```python
from build123d import *

# Parameters (mm, degrees)
SKETCH_1_W          = 15
SKETCH_1_H          = 15
SKETCH_1_W_2        = 12
SKETCH_1_H_2        = 12
EXTRUDE_1_DEPTH     = 220
SKETCH_2_R          = 1.6
CUT_EXTRUDE_1_DEPTH = 221.638278637
SKETCH_3_R          = 1.6
CUT_EXTRUDE_2_DEPTH = 221.638278637


with BuildPart() as part:
    # ｽｹｯﾁ1 → ﾎﾞｽ - 押し出し1 (new body)
    with BuildSketch(Plane(origin=(0, 0, 0), x_dir=(0, 0, -1), z_dir=(1, 0, 0))):
        Rectangle(SKETCH_1_W, SKETCH_1_H)
        Rectangle(SKETCH_1_W_2, SKETCH_1_H_2, mode=Mode.SUBTRACT)
    extrude(amount=EXTRUDE_1_DEPTH)

    # ｽｹｯﾁ2 → ｶｯﾄ - 押し出し1 (cut, through all)
    with BuildSketch(Plane(origin=(0, 7.5, 0), x_dir=(1, 0, 0), z_dir=(0, 1, 0))):
        with Locations(Location((66.961524227, 0, 0), (0, 0, 270))):
            Circle(SKETCH_2_R)
        with Locations(Location((45, 0, 0), (0, 0, 270))):
            Circle(SKETCH_2_R)
        with Locations(Location((175, 0, 0), (0, 0, 270))):
            Circle(SKETCH_2_R)
        with Locations(Location((153.038475773, 0, 0), (0, 0, 270))):
            Circle(SKETCH_2_R)
        with Locations(Location((22.5, 0, 0), (0, 0, 270))):
            Circle(SKETCH_2_R)
        with Locations(Location((197.5, 0, 0), (0, 0, 270))):
            Circle(SKETCH_2_R)
    extrude(amount=-CUT_EXTRUDE_1_DEPTH, mode=Mode.SUBTRACT)

    # ｽｹｯﾁ3 → ｶｯﾄ - 押し出し2 (cut, through all)
    with BuildSketch(Plane.XY.offset(7.5)):
        with Locations((7.5, 0)):
            Circle(SKETCH_3_R)
        with Locations((212.5, 0)):
            Circle(SKETCH_3_R)
    extrude(amount=-CUT_EXTRUDE_2_DEPTH, mode=Mode.SUBTRACT)


solid = part.part
```
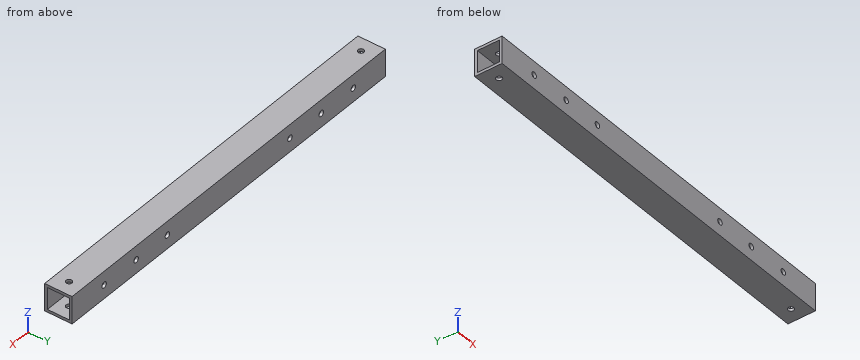
Here's how the part is built. I have some questions about the finished solid (model axes, mm). Round coordinates to 2 decimals unless told otherwise and drop trailing zeros. Loops run counter-clockwise (first coordinate to the right, second up) from the corner with the lowest first, then second, coordinate; pieces in that order, holes last.
1. If I drill on probe 1 along Z at (x, y) = (175, 6.95); probe 2 along Z at (x, y) = (22, -1.5), over which ranges is the centre line in solid material (lowest first)?
Answers:
probe 1: z = -7.5 to -1.6, 1.6 to 7.5
probe 2: z = -7.5 to -6, 6 to 7.5
2. Will this pin go through, and if not, where does the flat tip stop? pin 1 (3.5 mm diameter, centred on x = 197.5, z = 0, fed in from +Y).
Answers:
pin 1: stops at y = 7.5
3. Suppose I cut it at A-A, the plane x = 16.5. Please give me the cut outline in (y, z).
Answers:
outline: (-7.5, -7.5) - (7.5, -7.5) - (7.5, 7.5) - (-7.5, 7.5) - close; hole (-6, -6) - (6, -6) - (6, 6) - (-6, 6) - close
